Autodesk Inventor part; units mm, degrees
ref_plane "YZ Plane" through (0, 0, 0) normal (1, 0, 0) x (0, 1, 0)
ref_plane "XZ Plane" through (0, 0, 0) normal (0, 1, 0) x (-1, 0, 0)
ref_plane "XY Plane" through (0, 0, 0) normal (0, 0, 1) x (1, 0, 0)
ref_plane "Work Plane1" through (-43.5338, -0.5007, 1.2381) normal (0, 0, 1) x (1, 0, 0)
ref_plane "Work Plane2" through (-43.5338, -42.3785, -4.7563) normal (0, 0, 1) x (1, 0, 0)
sketch "Sketch1" plane through (-43.5338, -42.3785, -4.7563) normal (0, 0, 1) x (1, 0, 0)
  circle A0 centre (0, 41.8778) radius 4
  circle A1 centre (0, 0) radius 4
  circle A2 centre (0, -41.8778) radius 4
  circle A3 centre (-25.4, 41.8778) radius 2.54
  circle A4 centre (-25.3932, -41.7189) radius 2.54
  circle A5 centre (25.3979, 41.5493) radius 2.54
  circle A6 centre (25.8472, -41.7284) radius 2.54
  arc A7 (-24.8901, 51.9352) -> (-25.3932, 31.8075) centre (-25.4, 41.8778) ccw
  arc A8 (-25.3932, -31.3333) -> (-25.3932, -52.1046) centre (-25.3932, -41.7189) ccw
  arc A9 (25.4047, -52.1046) -> (35.6974, -38.4367) centre (25.8472, -41.7284) ccw
  arc A10 (35.7786, 41.8776) -> (25.3979, 51.9352) centre (25.3979, 41.5493) ccw
  line L0 (-24.8901, 51.9352) -> (25.3979, 51.9352)
  line L1 (35.7786, 41.8776) -> (22.8529, -0.0002)
  line L2 (22.8529, -0.0002) -> (35.6974, -38.4367)
  line L3 (25.4047, -52.1046) -> (-25.3932, -52.1046)
  line L4 (-25.3932, -31.3333) -> (-25.3932, 31.8075)
  point P0 (43.5338, 42.3785)
  dimension "d0" = 5.08
  dimension "d1" = 25.4
  dimension "d2" = 5.08
  dimension "d3" = 5.08
  dimension "d4" = 5.08
  dimension "d5" = 25.4
extrude "Extrusion1" add sketch "Sketch1" against normal blind 10
sketch "Sketch2" plane through (-43.5338, -42.3785, -14.7563) normal (0, 0, -1) x (-1, 0, 0)
  circle A0 centre (0, -41.8778) radius 4
  circle A1 centre (0, 0) radius 4
  circle A2 centre (0, 41.8778) radius 4
  circle A3 centre (-25.8472, -41.7284) radius 2.54
  circle A4 centre (-25.3979, 41.5493) radius 2.54
  circle A5 centre (25.3932, -41.7189) radius 2.54
  circle A6 centre (25.4, 41.8778) radius 2.54
  arc A7 (25.3932, 31.8075) -> (24.8901, 51.9352) centre (25.4, 41.8778) ccw
  line L0 (25.3932, 31.8075) -> (25.3932, -31.3333)
  arc A8 (25.3932, -52.1046) -> (25.3932, -31.3333) centre (25.3932, -41.7189) ccw
  line L1 (25.3932, -52.1046) -> (-25.4047, -52.1046)
  arc A9 (-35.6974, -38.4367) -> (-25.4047, -52.1046) centre (-25.8472, -41.7284) ccw
  line L2 (-35.6974, -38.4367) -> (-22.8529, -0.0002)
  line L3 (-22.8529, -0.0002) -> (-35.7786, 41.8776)
  arc A10 (-25.3979, 51.9352) -> (-35.7786, 41.8776) centre (-25.3979, 41.5493) ccw
  line L4 (-25.3979, 51.9352) -> (24.8901, 51.9352)
  circle A11 centre (0, 0) radius 11
  point P0 (-43.5338, 42.3785)
  dimension "d8" = 22
extrude "Extrusion2" cut sketch "Sketch2" against normal blind 8 contours A11
sketch "Sketch3" plane through (-43.5338, -42.3785, -4.7563) normal (0, 0, 1) x (1, 0, 0)
  circle A0 centre (0, 0) radius 5
  point P0 (43.5338, 42.3785)
  dimension "d11" = 10
extrude "Extrusion3" cut sketch "Sketch3" against normal blind 8
sketch "Sketch4" plane through (-43.5338, -42.3785, -14.7563) normal (0, 0, -1) x (-1, 0, 0)
  circle A0 centre (0, 0) radius 11
  circle A1 centre (0, -41.8778) radius 4
  circle A2 centre (0, 41.8778) radius 4
  circle A3 centre (-25.8472, -41.7284) radius 2.54
  circle A4 centre (-25.3979, 41.5493) radius 2.54
  circle A5 centre (25.3932, -41.7189) radius 2.54
  circle A6 centre (25.4, 41.8778) radius 2.54
  arc A7 (25.3932, 31.8075) -> (24.8901, 51.9352) centre (25.4, 41.8778) ccw
  line L0 (24.8901, 51.9352) -> (-25.3979, 51.9352)
  arc A8 (-25.3979, 51.9352) -> (-35.7786, 41.8776) centre (-25.3979, 41.5493) ccw
  line L1 (-35.7786, 41.8776) -> (-22.8529, -0.0002)
  line L2 (-22.8529, -0.0002) -> (-35.6974, -38.4367)
  arc A9 (-35.6974, -38.4367) -> (-25.4047, -52.1046) centre (-25.8472, -41.7284) ccw
  line L3 (-25.4047, -52.1046) -> (25.3932, -52.1046)
  arc A10 (25.3932, -52.1046) -> (25.3932, -31.3333) centre (25.3932, -41.7189) ccw
  line L4 (25.3932, -31.3333) -> (25.3932, 31.8075)
  line L5 (-19.5055, 3.4405) -> (-29.2362, 34.9666)
  arc A11 (-26.1883, -47.8914) -> (-25.5061, -47.8914) centre (-25.8472, -41.7284) ccw
  line L6 (-30.2853, -35.5342) -> (-19.5947, -3.5433)
  circle A12 centre (0, 41.8778) radius 4
  arc A13 (-29.2362, 34.9666) -> (-20.9299, 47.722) centre (-25.3979, 41.5493) ccw
  arc A14 (-21.366, -47.8914) -> (-30.2853, -35.5342) centre (-25.8472, -41.7284) ccw
  arc A15 (21.18, -35.3697) -> (20.925, -47.8914) centre (25.3932, -41.7189) ccw
  line L7 (-15.0962, 3.4405) -> (-19.5055, 3.4405)
  line L8 (-19.5947, -3.5433) -> (-15.0962, -3.5433)
  line L9 (21.18, 4.0176) -> (15.57, 4.0176)
  line L10 (15.6848, -3.5433) -> (21.18, -3.5433)
  line L11 (23.5004, 3.4405) -> (23.5004, 4.0176)
  line L12 (-2.4388, 15.894) -> (-2.4388, 33.1315)
  line L13 (1.6137, 32.9424) -> (1.6137, 15.9988)
  line L14 (-2.4388, -15.894) -> (-2.4388, -33.1315)
  line L15 (1.6137, -32.9424) -> (1.6137, -15.9988)
  line L16 (21.18, 35.533) -> (21.18, 4.0176)
  line L17 (21.18, -3.5433) -> (21.18, -37.208)
  arc A16 (20.5102, 47.722) -> (21.18, 35.533) centre (25.4, 41.8778) ccw
  line L18 (-20.9299, 47.722) -> (-6.9492, 47.722)
  line L19 (6.9492, 47.722) -> (20.5102, 47.722)
  arc A17 (15.57, 4.0176) -> (0.9078, 16.0544) centre (0, 0) ccw
  arc A18 (-2.4388, 15.894) -> (-15.7076, 3.4405) centre (0, 0) ccw
  arc A19 (-6.9492, 47.722) -> (-2.4388, 33.1315) centre (0, 41.8778) ccw
  arc A20 (1.6137, 32.9424) -> (6.9492, 47.722) centre (0, 41.8778) ccw
  arc A21 (-15.6848, -3.5433) -> (-1.8329, -15.9752) centre (0, 0) ccw
  arc A22 (0.9945, -16.0492) -> (15.6848, -3.5433) centre (0, 0) ccw
  arc A23 (-2.0453, -33.0312) -> (-6.8032, -47.8914) centre (0, -41.8778) ccw
  arc A24 (6.8032, -47.8914) -> (1.1925, -32.8765) centre (0, -41.8778) ccw
  line L20 (20.925, -47.8914) -> (6.8032, -47.8914)
  line L21 (-6.8032, -47.8914) -> (-21.366, -47.8914)
  point P0 (-43.5338, 42.3785)
  point P1 (18.8824, 0.2371)
  point P2 (-0.4126, 23.807)
  point P3 (-0.4126, -23.9098)
  dimension "d16" = 5.08
  dimension "d17" = 5.08
  dimension "d18" = 5.08
  dimension "d20" = 5.08
extrude "Extrusion4" cut sketch "Sketch4" against normal blind 6.5 contours L5 A13 L18 A19 L12 A18 L7 | L6 L8 A21 L14 A23 L21 A14 | A15 L20 A24 L15 A22 L10 L17 | L9 A17 L13 A20 L19 A16 L16
properties part number "Endstop"
Verification items for the finished model (mm, model axes). A direction names the side the tool comes from. Coordinates: 2 decimals unless noted, no trailing zeros. Loops run counter-clockwise (first coordinate to the right, second up) from the corner with the lowest first, then second, coordinate; pieces in that order, holes last. Notation, with made-up numbers: (73.5, 35) -> (102.5, 35) arc R7 ccw to (102.5, 43) -> close; hole circle Ø7 at (76, 66). An arc over 180 degrees is marked (long way). Answer in a Markdown table with one row per item. Add a question column.
1. Material ranges on probe 1 along Y at (x, z) = (-53.5, -10.5); probe 2 along Y at (x, z) = (-69, -8.5); probe 3 along X at (y, z) = (5, -11.5), recorded low to high. Write a range as [from, to].
2. Draft check along X on faces 3 (the face through (-18.52, -62.14, -11.55)), 4 (the face through (-10.83, 6.55, -9.69)), 5 (the face through (-43, -94.483, -10)). Enter one of: +X half, -X half, draft (parallel to the pull), parting line (faces both ways), or undercut.
3. Section check C-C, the plane z = -11. Give the number of separate pieces and of enclosed holes in the cut face, then the cut area to 3 significant figures.
4. Access from +Z, -Z, +X, -X, +Y, -Y to the whole of each face (thin tool, end or side, straight path). Record for faces 1 (the face through (-26, -38.938, -12)), 2 (the face through (-44, -30, -14.756)).
5. Section check D-D, the plane y = -13.5. Enter the section's corners in (x, z) (1 decimal), then the cut area to 3 significant figures.
6. Section check B-B, the plane y = -67. Enter the section's corners in (x, z) (1 decimal), then the cut area to 3 significant figures.
7. Depth check by flat-ended pin: P1, Ø2, axis at y = -70.5, z = -13, coming from the -X side; P2, Ø2, axis at x = -68.5, z = -7.5, coming from the -Y side; P3, Ø3, axis at y = -20.5, z = -10.5, coming from the +X side (3 decimals); P4, Ø3, axis at x = -18.14, y = -0.83, coming from the +Z side. Enter the tip coordinate at first touch or a pass-through.
8. Section check A-A, the plane y = -40.5. Enter the section's corners in (x, z).
Derived:
| question | item | result |
|---|---|---|
| 1 | probe 1 | y = [-94.48, -90.27], [-55, -47.03], [-37.72, -29.76], [5.34, 9.56] |
| 1 | probe 2 | y = [-94.48, -86.64], [-81.56, -73.71], [-10.57, -3.04], [2.04, 9.57] |
| 1 | probe 3 | x = [-77.37, -63.66], [-50.76, -36.31], [-23.04, -9.54] |
| 2 | face 3 | undercut |
| 2 | face 4 | +X half |
| 2 | face 5 | draft |
| 3 | separate pieces | 1 |
| 3 | enclosed holes | 11 |
| 3 | area | 2,910 mm² |
| 4 | face 1 | -Z |
| 4 | face 2 | -Z, +X, -X, +Y, -Y |
| 5 | outline | (-68.9, -14.8) -> (-64.7, -14.8) -> (-64.7, -8.3) -> (-45.1, -8.3) -> (-45.1, -14.8) -> (-41.1, -14.8) -> (-41.1, -8.3) -> (-16.2, -8.3) -> (-16.2, -14.8) -> (-11.8, -14.8) -> (-11.8, -4.8) -> (-68.9, -4.8) -> close |
| 5 | area | 282 mm² |
| 6 | outline | (-68.9, -14.8) -> (-64.7, -14.8) -> (-64.7, -8.3) -> (-45.1, -8.3) -> (-45.1, -14.8) -> (-41.1, -14.8) -> (-41.1, -8.3) -> (-16.9, -8.3) -> (-16.9, -14.8) -> (-12.5, -14.8) -> (-12.5, -4.8) -> (-68.9, -4.8) -> close |
| 6 | area | 280 mm² |
| 7 | P1 | stops at x = -68.93 |
| 7 | P2 | stops at y = -94.48 |
| 7 | P3 | stops at x = -13.465 |
| 7 | P4 | passes through |
| 8 | outline | (-68.93, -14.76) -> (-54.37, -14.76) -> (-54.37, -6.76) -> (-48.17, -6.76) -> (-48.17, -4.76) -> (-68.93, -4.76) -> close; (-38.9, -6.76) -> (-32.7, -6.76) -> (-32.7, -14.76) -> (-20.1, -14.76) -> (-20.1, -4.76) -> (-38.9, -4.76) -> close |
